```python
from build123d import *

# Parameters (mm, degrees)
BOSS_EXTRUDE1_DEPTH     = 11.7
SKETCH7_W               = 11.5
SKETCH7_H               = 0.65
CUT_EXTRUDE2_DEPTH      = 4
SKETCH7_4_R             = 1.6
BOSS_EXTRUDE2_DEPTH     = 1.4
CUT_EXTRUDE3_DEPTH      = 4.5
SKETCH7_6_R             = 1.85
CUT_EXTRUDE4_DEPTH      = 2.4
CUT_EXTRUDE4_DEPTH_BACK = 10.7
CUT_EXTRUDE5_DEPTH      = 3
SKETCH12_W              = 1.5
SKETCH12_H              = 21.000689182
CUT_EXTRUDE6_DEPTH      = 3
SKETCH14_W              = 2.2
SKETCH14_H              = 4
BOSS_EXTRUDE3_DEPTH     = 1
FILLET3_R               = 1.5
FILLET4_R               = 0.25


with BuildPart() as part:
    # Sketch1 → Boss-Extrude1 (new body)
    with BuildSketch(Plane(origin=(0, 0, 0), x_dir=(1, 0, 0), z_dir=(0, 1, 0))):
        Polygon((-28.77817965, 14.04419618), (-24.27817965, 14.04419618), (-24.27817965, 22.04419618), (-22.07817965, 22.04419618), (-22.07817965, 14.04419618), (-19.07817965, 14.04419618), (-19.07817965, 2.54419618), (-28.77817965, 2.54419618), align=None)
    extrude(amount=BOSS_EXTRUDE1_DEPTH)

    # Sketch7 → Cut-Extrude2 (cut)
    with BuildSketch(Plane.ZY.offset(28.77817965)):
        with Locations((-8.29419618, 10.875)):
            Rectangle(SKETCH7_W, SKETCH7_H)
    extrude(amount=-CUT_EXTRUDE2_DEPTH, mode=Mode.SUBTRACT)

    # Sketch7<4> → Boss-Extrude2 (add)
    with BuildSketch(Plane.ZY.offset(28.77817965)):
        with Locations((-10.79419618, 8.2)):
            Circle(SKETCH7_4_R)
    extrude(amount=BOSS_EXTRUDE2_DEPTH)

    # Sketch7<5> → Cut-Extrude3 (cut)
    with BuildSketch(Plane.ZY.offset(28.77817965)):
        Polygon((-2.54419618, 0.097302003), (-14.04419618, 8.2), (-14.04419618, 0), (-2.54419618, 0), align=None)
    extrude(amount=-CUT_EXTRUDE3_DEPTH, mode=Mode.SUBTRACT)

    # Sketch7<6> → Cut-Extrude4 (cut, two sides)
    with BuildSketch(Plane.ZY.offset(28.77817965)) as cut_extrude4_sk:
        with Locations((-18.04419618, 9.2)):
            Circle(SKETCH7_6_R)
    extrude(amount=CUT_EXTRUDE4_DEPTH, mode=Mode.SUBTRACT)
    extrude(cut_extrude4_sk.sketch, amount=-CUT_EXTRUDE4_DEPTH_BACK, mode=Mode.SUBTRACT)

    # Sketch10 → Cut-Extrude5 (cut)
    with BuildSketch(Plane(origin=(-22.07817965, 0, 0), x_dir=(0, 0, -1), z_dir=(1, 0, 0))):
        Polygon((15.54419618, 9.2), (15.54419618, 0), (2.54419618, 0), (2.54419618, 0.097302003), align=None)
    extrude(amount=CUT_EXTRUDE5_DEPTH, mode=Mode.SUBTRACT)

    # Sketch12 → Cut-Extrude6 (cut)
    with BuildSketch(Plane.XZ):
        with Locations((-23.17817965, -11.543851589)):
            Rectangle(SKETCH12_W, SKETCH12_H)
    extrude(amount=-CUT_EXTRUDE6_DEPTH, mode=Mode.SUBTRACT)

    # Sketch14 → Boss-Extrude3 (add)
    with BuildSketch(Plane(origin=(0, 0, 0), x_dir=(-1, 0, 0), z_dir=(0, -1, 0))):
        with Locations((23.17817965, 4.54419618)):
            Rectangle(SKETCH14_W, SKETCH14_H)
    extrude(amount=-BOSS_EXTRUDE3_DEPTH)

    # Fillet3
    fillet3_edges = [part.edges().sort_by_distance(p)[0] for p in [
        (-26.52817965, 8.2, -14.04419618),
        (-20.57817965, 8.149688693, -14.04419618),
        (-26.52817965, 11.7, -14.04419618),
        (-20.57817965, 11.7, -14.04419618),
        (-19.07817965, 4.123495348, -8.29419618),
        (-19.07817965, 9.924844346, -14.04419618),
        (-19.07817965, 11.7, -8.29419618),
        (-23.17817965, 11.7, -22.04419618),
        (-24.10317965, 0, -22.04419618),
        (-22.25317965, 0, -22.04419618),
    ]]
    fillet(fillet3_edges, radius=FILLET3_R)

    # Mirror3: part across plane


with BuildPart() as part_1:
    add(part.part)
    add(part.part.mirror(Plane(origin=(-19.07817965, 11.7, -2.54419618), x_dir=(1, 0, 0), z_dir=(0, 0, -1))))

    # Fillet4
    fillet4_edges = [part_1.edges().sort_by_distance(p)[0] for p in [
        (-22.42817965, 3, -2.54419618),
        (-23.92817965, 3, -2.54419618),
        (-23.92817965, 2.25, -22.04419618),
        (-23.17817965, 3, -22.04419618),
        (-22.42817965, 2.25, -22.04419618),
        (-23.92817965, 0, -13.54419618),
        (-23.92817965, 1, -2.54419618),
        (-23.92817965, 0.5, -6.54419618),
        (-23.17817965, 1, -6.54419618),
        (-22.42817965, 0.5, -6.54419618),
        (-22.42817965, 1, -2.54419618),
        (-23.17817965, 0, -6.54419618),
        (-22.42817965, 0, -13.54419618),
        (-23.92817965, 0.439339828, -21.604856352),
        (-22.42817965, 0.439339828, -21.604856352),
        (-24.77817965, 10.55, -2.54419618),
        (-23.17817965, 3, 16.95580382),
        (-22.42817965, 2.25, 16.95580382),
        (-22.42817965, 0, 8.45580382),
        (-23.92817965, 0, 8.45580382),
        (-23.92817965, 2.25, 16.95580382),
        (-22.42817965, 0.5, 1.45580382),
        (-23.92817965, 0.5, 1.45580382),
        (-23.17817965, 0, 1.45580382),
        (-23.17817965, 1, 1.45580382),
        (-23.92817965, 0.439339828, 16.516463992),
        (-22.42817965, 0.439339828, 16.516463992),
        (-24.77817965, 11.2, -2.54419618),
    ]]
    fillet(fillet4_edges, radius=FILLET4_R)


solid = part_1.part
```
Geometry check sheet. Reference: the model listing, model coordinates, mm. A direction names the side the tool comes from. Give positions to 0.01 mm unless a question says otherwise; leave off trailing zeros. Loops run counter-clockwise (first coordinate to the right, second up) from the corner with the lowest first, then second, coordinate; pieces in that order, holes last. Notation, with made-up numbers: M -3,-38 L 6,-38 A15 cw 6,-18 Z; hole C -29,-7 d2. An arc over 180 degrees is marked long. Write item = value, one per line.
(1) Sectioned sample at C-C, the plane y = 8.2. State how many separate pieces and enclosed holes the cut face has, plus the area to 3 significant figures.
Answer below:
separate_pieces = 3
enclosed_holes = 0
area = 249 mm2
(2) Sectioned sample at A-A, the plane x = -27. Record the cut outline in (y, z), plus the area to 3 significant figures.
Answer below:
outline = M 0.1,-2.54 L 7.75,-13.41 A1.5 ccw 8.98,-14.04 L 10.2,-14.04 A1.5 ccw 10.55,-14 L 10.55,8.91 A1.5 ccw 10.2,8.96 L 8.98,8.96 A1.5 ccw 7.75,8.32 Z; M 11.2,-13.66 A1.5 ccw 11.7,-12.54 L 11.7,7.46 A1.5 ccw 11.2,8.57 Z
area = 158 mm2
(3) Tool access check on faces 4 (the face through (-21.318, 11.272, 8.505)), 5 (the face through (-27, 10.55, -2)), 6 (the face through (-21.318, 11.272, -13.593)), 7 (the face through (-26.56, 3.87, 2.81)). Record the directions out of +Z, -Z, +X, -X, +Y, -Y that give a thin tool (end or side, any length) a straight path to the whole face; none if there is none.
Answer below:
face_4 = +Z, +X, +Y
face_5 = +Z, -Z, -X
face_6 = -Z, +X, +Y
face_7 = +Z, -X, -Y
(4) Gauge pin test, flat ends, axial feed: pin 1 Ø1.5 at (x, z) = (-26, 10) entering from -Y; pin 2 Ø0.6 at (y, z) = (11.5, -7) entering from -X; pin 3 Ø1.1 at (x, z) = (-26.5, -6.5) entering from -Y; pin 4 Ø3 at (x, y) = (-27.5, 1.5) entering from -Z. Record the tip position at first contact, or that the pin passes through.
Answer below:
pin_1 = through
pin_2 = -28.78
pin_3 = 2.5
pin_4 = -6.66
(5) Release check for a two-part mould opening along X. For faces 1 (the face through (-23, 7, -22.044)), 2 (the face through (-19.5, 9.6, 8.5)), 3 (the face through (-23, 1, -2)) record: released by +X, released by -X, zero draft, split by the parting line, or undercut.
Answer below:
face_1 = zero draft
face_2 = released by +X
face_3 = undercut
(6) Material ranges on line 1 (X direction, y = 2.25, z = 13.5); line 2 (X direction, y = 4.75, z = 10.5); line 3 (Y direction, x = -27, z = -13.5), recorded low to high. Write a range as [from, to].
Answer below:
line_1 = [-24.28, -23.93], [-22.43, -22.08]
line_2 = [-24.28, -22.08]
line_3 = [7.82, 10.55], [11.2, 11.36]
(7) Sectioned sample at B-B, the plane z = 10.5. Record the cut outline in (x, y), plus the area to 3 significant figures.
Answer below:
outline = M -24.28,0 L -24.18,0 A0.25 ccw -23.93,0.25 L -23.93,2.75 A0.25 cw -23.68,3 L -22.68,3 A0.25 cw -22.43,2.75 L -22.43,0.25 A0.25 ccw -22.18,0 L -22.08,0 L -22.08,11.7 L -24.28,11.7 Z
area = 21.2 mm2
